```python
from build123d import *

# Parameters (mm, degrees)
SKETCH_2_W          = 807
SKETCH_2_H          = 307
EXTRUDE_1_DEPTH     = 25
SKETCH_3_W          = 801
SKETCH_3_H          = 301
CUT_EXTRUDE_1_DEPTH = 22
SKETCH_4_R          = 3
CUT_EXTRUDE_2_DEPTH = 308
SKETCH_5_R          = 60
CUT_EXTRUDE_3_DEPTH = 26


with BuildPart() as part:
    # 草圖2 → 填料-伸長1 (new body)
    with BuildSketch(Plane(origin=(0, 0, 0), x_dir=(1, 0, 0), z_dir=(0, 1, 0))):
        with Locations((403.5, -153.5)):
            Rectangle(SKETCH_2_W, SKETCH_2_H)
    extrude(amount=EXTRUDE_1_DEPTH)

    # 草圖3 → 除料-伸長1 (cut)
    with BuildSketch(Plane(origin=(0, 25, 0), x_dir=(1, 0, 0), z_dir=(0, 1, 0))):
        with Locations((403.5, -153.5)):
            Rectangle(SKETCH_3_W, SKETCH_3_H)
    extrude(amount=-CUT_EXTRUDE_1_DEPTH, mode=Mode.SUBTRACT)

    # 草圖4 → 除料-伸長2 (cut, through all)
    with BuildSketch(Plane.XY.offset(307)):
        with Locations((759, 12.5)):
            Circle(SKETCH_4_R)
        with Locations((48, 12.5)):
            Circle(SKETCH_4_R)
    extrude(amount=-CUT_EXTRUDE_2_DEPTH, mode=Mode.SUBTRACT)

    # 草圖5 → 除料-伸長3 (cut, through all)
    with BuildSketch(Plane.XZ):
        with Locations((607, 207)):
            Circle(SKETCH_5_R)
        with Locations((200, 207)):
            Circle(SKETCH_5_R)
    extrude(amount=-CUT_EXTRUDE_3_DEPTH, mode=Mode.SUBTRACT)


solid = part.part
```
Verification items for the finished model (mm, model axes). A direction names the side the tool comes from. Give positions to 0.01 mm unless a question says otherwise; leave off trailing zeros. Loops run counter-clockwise (first coordinate to the right, second up) from the corner with the lowest first, then second, coordinate; pieces in that order, holes last. Notation, with made-up numbers: M 75,30 L 100,30 A32 cw 100,67 Z; hole C 25,75 d2. An arc over 180 degrees is marked long. Return JSON: item names as keys, results as strings.
1) Material ranges on L1, parallel to Z at x = 295, y = 21.5; L2, parallel to Z at x = 607, y = 1.5; L3, parallel to X at y = 11.75, z = 183.5, recorded low to high. Write a range as [from, to].
Findings:
{"L1": "z = [0, 3], [304, 307]", "L2": "z = [0, 147], [267, 307]", "L3": "x = [0, 3], [804, 807]"}
2) Tool access check on faces 1 (the cylindrical face through (547.06, 1.48, 209.64)), 2 (the flat face through (398, 14, 3)). Record the directions out of +Z, -Z, +X, -X, +Y, -Y that give a thin tool (end or side, any length) a straight path to the whole face; none if there is none.
Findings:
{"face 1": "+Y, -Y", "face 2": "+Y"}
3) Section check A-A, the plane z = 207. Enter the section's corners in (x, y), and give its area (3 significant figures).
Findings:
{"outline": "M 0,0 L 140,0 L 140,3 L 3,3 L 3,25 L 0,25 Z; M 260,0 L 547,0 L 547,3 L 260,3 Z; M 667,0 L 807,0 L 807,25 L 804,25 L 804,3 L 667,3 Z", "area": "1,830 mm2"}
4) Section check B-B, the plane x = 607. Enter the section's corners in (y, z), and give its area (3 significant figures).
Findings:
{"outline": "M 0,0 L 25,0 L 25,3 L 3,3 L 3,147 L 0,147 Z; M 0,267 L 3,267 L 3,304 L 25,304 L 25,307 L 0,307 Z", "area": "693 mm2"}
5) Section check C-C, the plane y = 20.75. Enter the section's corners in (x, z), and give its area (3 significant figures).
Findings:
{"outline": "M 0,0 L 807,0 L 807,307 L 0,307 Z; hole M 3,3 L 804,3 L 804,304 L 3,304 Z", "area": "6,650 mm2"}
6) Mould release check, pull along X, two halves, no side actions. Record for faces 3 (the flat face through (398, 12, 0)), 4 (the flat face through (807, 12, 156)), 5 (the flat face through (0, 12, 156)), 6 (the flat face through (398, 3, 151)): released by +X, released by -X, zero draft, split by the parting line, or undercut.
Findings:
{"face 3": "zero draft", "face 4": "released by +X", "face 5": "released by -X", "face 6": "undercut"}
7) Section check D-D, the plane z = 21. Enter the section's corners in (x, y), and give its area (3 significant figures).
Findings:
{"outline": "M 0,0 L 807,0 L 807,25 L 804,25 L 804,3 L 3,3 L 3,25 L 0,25 Z", "area": "2,550 mm2"}
8) Gauge pin test, flat ends, axial feed: P1, Ø11, axis at y = 15, z = 100, coming from the -X side; P2, Ø12, axis at x = 354, z = 268, coming from the +Y side. Record the tip position at first contact, or that the pin passes through.
Findings:
{"P1": "stops at x = 0", "P2": "stops at y = 3"}
